For this review, use the dimensioned drawing (mm, ordinates from the lowest corner) and the shaded views. A direction names the side the tool comes from. Give positions to 0.01 mm unless a question says otherwise; leave off trailing zeros. Write each loop counter-clockwise with the first axis right and the second up, starting at its lowest first coordinate (ties: lowest second). Pieces come first, ordered by that corner, then holes. Notation, with made-up numbers: M -36,29.5 L 5,29.5 A14 ccw 5,43.5 Z; hole C 51,-16.5 d3. An arc over 180 degrees is marked long. Use a Markdown table: item, result. Add a question column.
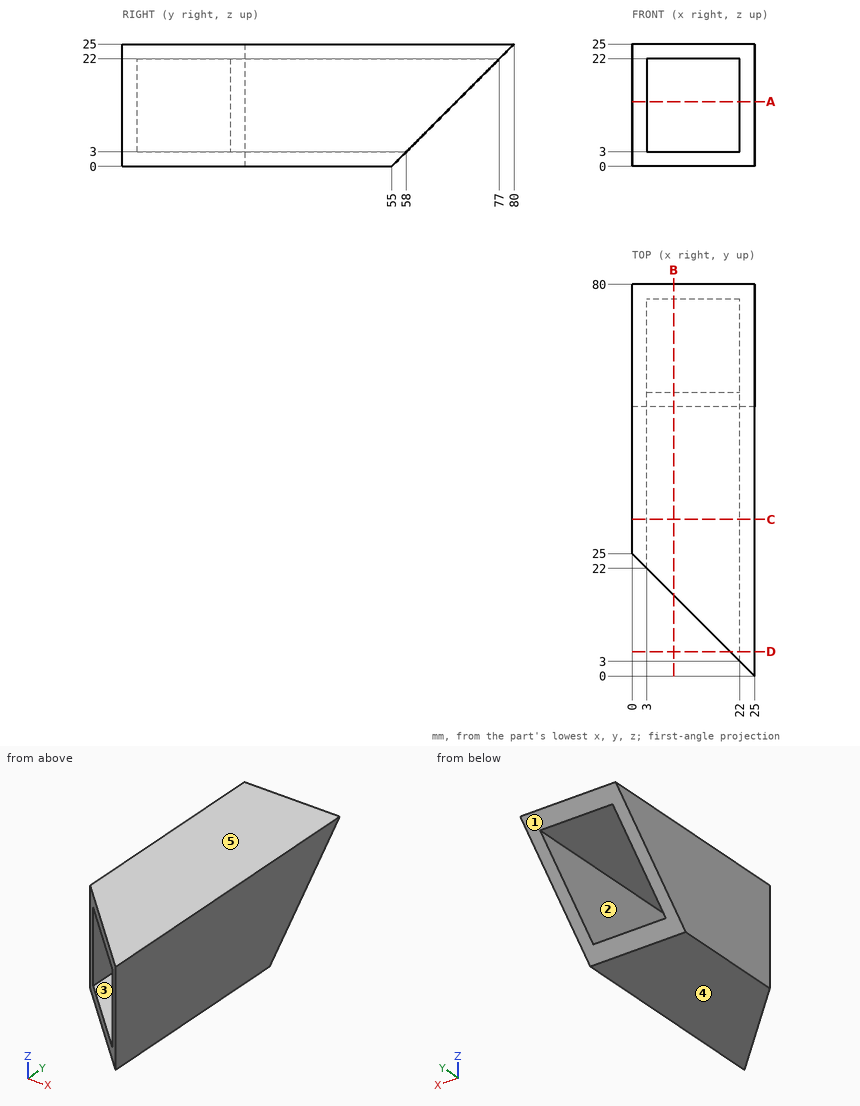
(1) Add section D-D on y = 5. Give the boundary of the cut face in (x, z).
(2) Add section A-A on z = 13.25. Give the boundary of the cut face in (x, y), then the cut area to 4 significant figures.
(3) Machinability: for the marked faces 1 and 2, which of the approach directions +Z, -Z, +X, -X, +Y, -Y give a long, thin tool a straight path to every point of the face, cutting with its end or side? Answer none if there is none.
(4) The part is to be moulded in two halves that separate along Z. For the marked faces 3, 4 and 5, say which applies: released by +Z, released by -Z, zero draft, split by the parting line, or undercut.
(5) Wall thickness on L1, parallel to Z at x = 10.75, y = 35.5; L2, parallel to X at y = 6, z = 21: over which ranges is each line inside the solid? List them lowest first.
(6) Add section C-C on y = 32. Give the boundary of the cut face in (x, z), then the cut area to 3 significant figures.
(7) Add section B-B on x = 8.5. Give the boundary of the cut face in (y, z), then the cut area to 3 significant figures.
From the geometry:
| question | item | result |
|---|---|---|
| 1 | outline | M 20,0 L 25,0 L 25,25 L 20,25 L 20,22 L 22,22 L 22,3 L 20,3 Z |
| 2 | outline | M 0,25 L 3,22 L 3,68.25 L 0,68.25 Z; M 22,3 L 25,0 L 25,68.25 L 22,68.25 Z |
| 2 | area | 334.5 mm^2 |
| 3 | face 1 | -Z, +X, -X, +Y |
| 3 | face 2 | +Y, -Y |
| 4 | face 3 | undercut |
| 4 | face 4 | released by -Z |
| 4 | face 5 | released by +Z |
| 5 | L1 | z = 0 to 3, 22 to 25 |
| 5 | L2 | x = 22 to 25 |
| 6 | outline | M 0,0 L 25,0 L 25,25 L 0,25 Z; hole M 3,3 L 22,3 L 22,22 L 3,22 Z |
| 6 | area | 264 mm^2 |
| 7 | outline | M 16.5,0 L 55,0 L 58,3 L 16.5,3 Z; M 16.5,22 L 77,22 L 80,25 L 16.5,25 Z |
| 7 | area | 306 mm^2 |
